from build123d import *

# Parameters (mm, degrees)
F1_DEPTH = 22.86
F2_R     = 10.16
F3_DEPTH = 38.1


with BuildPart() as f1:
    # F0 (on Right) → F1 (new body)
    with BuildSketch(Plane.YZ):
        with BuildLine():
            Line((23.650777, 0), (25.379719, 1.014815))
            Line((25.379719, 1.014815), (23.650777, 1.661146))
            Line((23.650777, 1.661146), (25.290415, 2.356882))
            Line((25.290415, 2.356882), (23.538487, 3.094504))
            Line((23.538487, 3.094504), (25.025895, 4.343339))
            Line((25.025895, 4.343339), (22.934098, 4.803507))
            Line((22.934098, 4.803507), (24.565468, 6.457382))
            Line((24.565468, 6.457382), (22.934098, 6.457382))
            Line((22.934098, 6.457382), (24.051407, 8.166384))
            Line((24.051407, 8.166384), (22.437936, 8.166384))
            Line((22.437936, 8.166384), (23.538487, 9.544612))
            Line((23.538487, 9.544612), (21.677369, 9.544612))
            Line((21.677369, 9.544612), (22.743621, 11.308745))
            Line((22.743621, 11.308745), (20.61609, 11.308745))
            Line((20.61609, 11.308745), (21.677369, 13.238265))
            Line((21.677369, 13.238265), (19.791737, 13.238265))
            Line((19.791737, 13.238265), (20.61609, 14.837009))
            Line((20.61609, 14.837009), (18.285365, 14.837009))
            Line((18.285365, 14.837009), (19.237809, 16.585135))
            Line((19.237809, 16.585135), (17.33292, 15.836925))
            Line((17.33292, 15.836925), (17.33292, 18.566903))
            Line((17.33292, 18.566903), (15.356795, 17.790713))
            Line((15.356795, 17.790713), (15.356795, 20.231877))
            Line((15.356795, 20.231877), (13.300184, 19.424073))
            Line((13.300184, 19.424073), (13.300184, 21.639434))
            Line((13.300184, 21.639434), (11.304469, 20.85555))
            Line((11.304469, 20.85555), (11.304469, 22.745746))
            Line((11.304469, 22.745746), (9.314078, 21.963953))
            Line((9.314078, 21.963953), (9.314078, 23.630657))
            Line((9.314078, 23.630657), (7.061159, 22.745746))
            Line((7.061159, 22.745746), (7.061159, 24.398771))
            Line((7.061159, 24.398771), (5.105594, 23.630657))
            Line((5.105594, 23.630657), (5.105594, 24.881578))
            Line((5.105594, 24.881578), (3.804288, 23.933317))
            Line((3.804288, 23.933317), (2.852615, 25.239306))
            Line((2.852615, 25.239306), (2.095285, 23.933317))
            Line((2.095285, 23.933317), (1.213507, 25.370995))
            ThreePointArc((1.213507, 25.370995), (1.101785, 25.376093), (0.990041, 25.380698))
            Line((0.990041, 25.380698), (0, 23.933317))
            Line((0, 23.933317), (-1.213507, 25.370995))
            Line((-1.213507, 25.370995), (-2.095285, 23.933317))
            Line((-2.095285, 23.933317), (-2.852615, 25.239306))
            Line((-2.852615, 25.239306), (-3.804288, 23.933317))
            Line((-3.804288, 23.933317), (-5.105594, 24.881578))
            Line((-5.105594, 24.881578), (-5.105594, 23.630657))
            Line((-5.105594, 23.630657), (-7.061159, 24.398771))
            Line((-7.061159, 24.398771), (-7.061159, 22.745746))
            Line((-7.061159, 22.745746), (-9.314078, 23.630657))
            Line((-9.314078, 23.630657), (-9.314078, 21.963953))
            Line((-9.314078, 21.963953), (-11.304469, 22.745746))
            Line((-11.304469, 22.745746), (-11.304469, 20.85555))
            Line((-11.304469, 20.85555), (-13.300184, 21.639434))
            Line((-13.300184, 21.639434), (-13.300184, 19.424073))
            Line((-13.300184, 19.424073), (-15.356795, 20.231877))
            Line((-15.356795, 20.231877), (-15.356795, 17.790713))
            Line((-15.356795, 17.790713), (-17.33292, 18.566903))
            Line((-17.33292, 18.566903), (-17.33292, 15.836925))
            Line((-17.33292, 15.836925), (-19.237809, 16.585135))
            Line((-19.237809, 16.585135), (-18.285365, 14.837009))
            Line((-18.285365, 14.837009), (-20.61609, 14.837009))
            Line((-20.61609, 14.837009), (-19.791737, 13.238265))
            Line((-19.791737, 13.238265), (-21.677369, 13.238265))
            Line((-21.677369, 13.238265), (-20.61609, 11.308745))
            Line((-20.61609, 11.308745), (-22.743621, 11.308745))
            Line((-22.743621, 11.308745), (-21.677369, 9.544612))
            Line((-21.677369, 9.544612), (-23.538487, 9.544612))
            Line((-23.538487, 9.544612), (-22.437936, 8.166384))
            Line((-22.437936, 8.166384), (-24.051407, 8.166384))
            Line((-24.051407, 8.166384), (-22.934098, 6.457382))
            Line((-22.934098, 6.457382), (-24.565468, 6.457382))
            Line((-24.565468, 6.457382), (-22.934098, 4.803507))
            Line((-22.934098, 4.803507), (-25.025895, 4.343339))
            Line((-25.025895, 4.343339), (-23.538487, 3.094504))
            Line((-23.538487, 3.094504), (-25.290415, 2.356882))
            Line((-25.290415, 2.356882), (-23.650777, 1.661146))
            Line((-23.650777, 1.661146), (-25.379719, 1.014815))
            Line((-25.379719, 1.014815), (-23.650777, 0))
            Line((-23.650777, 0), (-25.290127, -1.048307))
            Line((-25.290127, -1.048307), (-23.650777, -1.661146))
            Line((-23.650777, -1.661146), (-25.290415, -2.356882))
            Line((-25.290415, -2.356882), (-23.538487, -3.094504))
            Line((-23.538487, -3.094504), (-25.025895, -4.343339))
            Line((-25.025895, -4.343339), (-22.934098, -4.803507))
            Line((-22.934098, -4.803507), (-24.565468, -6.457382))
            Line((-24.565468, -6.457382), (-22.934098, -6.457382))
            Line((-22.934098, -6.457382), (-24.051407, -8.166384))
            Line((-24.051407, -8.166384), (-22.437936, -8.166384))
            Line((-22.437936, -8.166384), (-23.538487, -9.544612))
            Line((-23.538487, -9.544612), (-21.677369, -9.544612))
            Line((-21.677369, -9.544612), (-22.743621, -11.308745))
            Line((-22.743621, -11.308745), (-20.61609, -11.308745))
            Line((-20.61609, -11.308745), (-21.677369, -13.238265))
            Line((-21.677369, -13.238265), (-19.791737, -13.238265))
            Line((-19.791737, -13.238265), (-20.61609, -14.837009))
            Line((-20.61609, -14.837009), (-18.285365, -14.837009))
            Line((-18.285365, -14.837009), (-19.237809, -16.585135))
            Line((-19.237809, -16.585135), (-17.33292, -15.836925))
            Line((-17.33292, -15.836925), (-17.33292, -18.566903))
            Line((-17.33292, -18.566903), (-15.356795, -17.790713))
            Line((-15.356795, -17.790713), (-15.356795, -20.231877))
            Line((-15.356795, -20.231877), (-13.300184, -19.424073))
            Line((-13.300184, -19.424073), (-13.300184, -21.639434))
            Line((-13.300184, -21.639434), (-11.304469, -20.85555))
            Line((-11.304469, -20.85555), (-11.304469, -22.745746))
            Line((-11.304469, -22.745746), (-9.314078, -21.963953))
            Line((-9.314078, -21.963953), (-9.314078, -23.630657))
            Line((-9.314078, -23.630657), (-7.061159, -22.745746))
            Line((-7.061159, -22.745746), (-7.061159, -24.398771))
            Line((-7.061159, -24.398771), (-5.105594, -23.630657))
            Line((-5.105594, -23.630657), (-5.105594, -24.881578))
            Line((-5.105594, -24.881578), (-3.804288, -23.933317))
            Line((-3.804288, -23.933317), (-2.852615, -25.239306))
            Line((-2.852615, -25.239306), (-2.095285, -23.933317))
            Line((-2.095285, -23.933317), (-1.213507, -25.370995))
            Line((-1.213507, -25.370995), (0, -23.933317))
            Line((0, -23.933317), (0.990041, -25.380698))
            ThreePointArc((0.990041, -25.380698), (1.101785, -25.376093), (1.213507, -25.370995))
            Line((1.213507, -25.370995), (2.095285, -23.933317))
            Line((2.095285, -23.933317), (2.852615, -25.239306))
            Line((2.852615, -25.239306), (3.804288, -23.933317))
            Line((3.804288, -23.933317), (5.105594, -24.881578))
            Line((5.105594, -24.881578), (5.105594, -23.630657))
            Line((5.105594, -23.630657), (7.061159, -24.398771))
            Line((7.061159, -24.398771), (7.061159, -22.745746))
            Line((7.061159, -22.745746), (9.314078, -23.630657))
            Line((9.314078, -23.630657), (9.314078, -21.963953))
            Line((9.314078, -21.963953), (11.304469, -22.745746))
            Line((11.304469, -22.745746), (11.304469, -20.85555))
            Line((11.304469, -20.85555), (13.300184, -21.639434))
            Line((13.300184, -21.639434), (13.300184, -19.424073))
            Line((13.300184, -19.424073), (15.356795, -20.231877))
            Line((15.356795, -20.231877), (15.356795, -17.790713))
            Line((15.356795, -17.790713), (17.33292, -18.566903))
            Line((17.33292, -18.566903), (17.33292, -15.836925))
            Line((17.33292, -15.836925), (19.237809, -16.585135))
            Line((19.237809, -16.585135), (18.285365, -14.837009))
            Line((18.285365, -14.837009), (20.61609, -14.837009))
            Line((20.61609, -14.837009), (19.791737, -13.238265))
            Line((19.791737, -13.238265), (21.677369, -13.238265))
            Line((21.677369, -13.238265), (20.61609, -11.308745))
            Line((20.61609, -11.308745), (22.743621, -11.308745))
            Line((22.743621, -11.308745), (21.677369, -9.544612))
            Line((21.677369, -9.544612), (23.538487, -9.544612))
            Line((23.538487, -9.544612), (22.437936, -8.166384))
            Line((22.437936, -8.166384), (24.051407, -8.166384))
            Line((24.051407, -8.166384), (22.934098, -6.457382))
            Line((22.934098, -6.457382), (24.565468, -6.457382))
            Line((24.565468, -6.457382), (22.934098, -4.803507))
            Line((22.934098, -4.803507), (25.025895, -4.343339))
            Line((25.025895, -4.343339), (23.538487, -3.094504))
            Line((23.538487, -3.094504), (25.290415, -2.356882))
            Line((25.290415, -2.356882), (23.650777, -1.661146))
            Line((23.650777, -1.661146), (25.290127, -1.048307))
            Line((25.290127, -1.048307), (23.650777, 0))
        make_face()
    extrude(amount=F1_DEPTH)

    # F2 (on face) → F3 (cut)
    with BuildSketch(Plane.YZ.offset(22.86)):
        Circle(F2_R)
    extrude(amount=-F3_DEPTH, mode=Mode.SUBTRACT)


solid = f1.part
Verification items for the finished model (mm, model axes). A direction names the side the tool comes from. Give positions to 0.01 mm unless a question says otherwise; leave off trailing zeros. Write each loop counter-clockwise with the first axis right and the second up, starting at its lowest first coordinate (ties: lowest second). Pieces come first, ordered by that corner, then holes. Notation, with made-up numbers: (-17, 69.25) - (30, 69.25) arc R25 cw to (30, 83.25) - close; hole circle Ø6 at (83, -19.5). An arc over 180 degrees is marked (long way). Answer as CSV lines item,"result". Start each with the question number.
1. Thickness scan on line 1 (Y direction, x = 20, z = 5.5); line 2 (Y direction, x = 9.25, z = -5); line 3 (Y direction, x = 11.75, z = 17). Record the ranges inside material, lowest first.
2. Depth check by flat-ended pin: pin 1 (0.6 mm diameter, centred on x = 15, y = 21.5, fed in from +Z); pin 2 (0.9 mm diameter, centred on x = 10.5, z = -21.5, fed in from -Y); pin 3 (12 mm diameter, centred on x = 13.5, y = -14, fed in from +Z). Enter the tip coordinate at first touch or a pass-through.
3. Draft check along Z on faces 1 (the face through (11.27, -14.343, -19.834)), 2 (the face through (11, 22, 11.309)), 3 (the face through (11.27, 14.343, 19.834)), 4 (the face through (11.27, 23.485, 7.3)). Enter one of: pulls with the +Z half, pulls with the -Z half, needs draft (parallel to the pull), parting line crosses it, or undercut.
4. Sectioned sample at A-A (y = -6). Record the boundary of the cut face in (x, z), then the cut area to 3 significant figures.
5. Set-up check for faces 5 (the face through (11.27, -12.288, 21.242)), 6 (the face through (11.27, 0.49, -24.65)): record each of +Z, -Z, +X, -X, +Y, -Y from which the full face is reachable in a straight line by a thin tool's end or side.
Derived:
1,line 1,"-23.62 to -8.54, 8.54 to 23.62"
1,line 2,"-23.13 to -8.84, 8.84 to 23.13"
1,line 3,"-17.33 to 17.33"
2,pin 1,"z = 13.24"
2,pin 2,"y = -13.3"
2,pin 3,"z = 23.63"
3,face 1,"pulls with the -Z half"
3,face 2,"undercut"
3,face 3,"pulls with the +Z half"
3,face 4,"undercut"
4,outline,"(0, -23.98) - (22.86, -23.98) - (22.86, -8.2) - (0, -8.2) - close; (0, 8.2) - (22.86, 8.2) - (22.86, 23.98) - (0, 23.98) - close"
4,area,"722 mm²"
5,face 5,"+Z, +X, -X"
5,face 6,"-Z, +X, -X"
